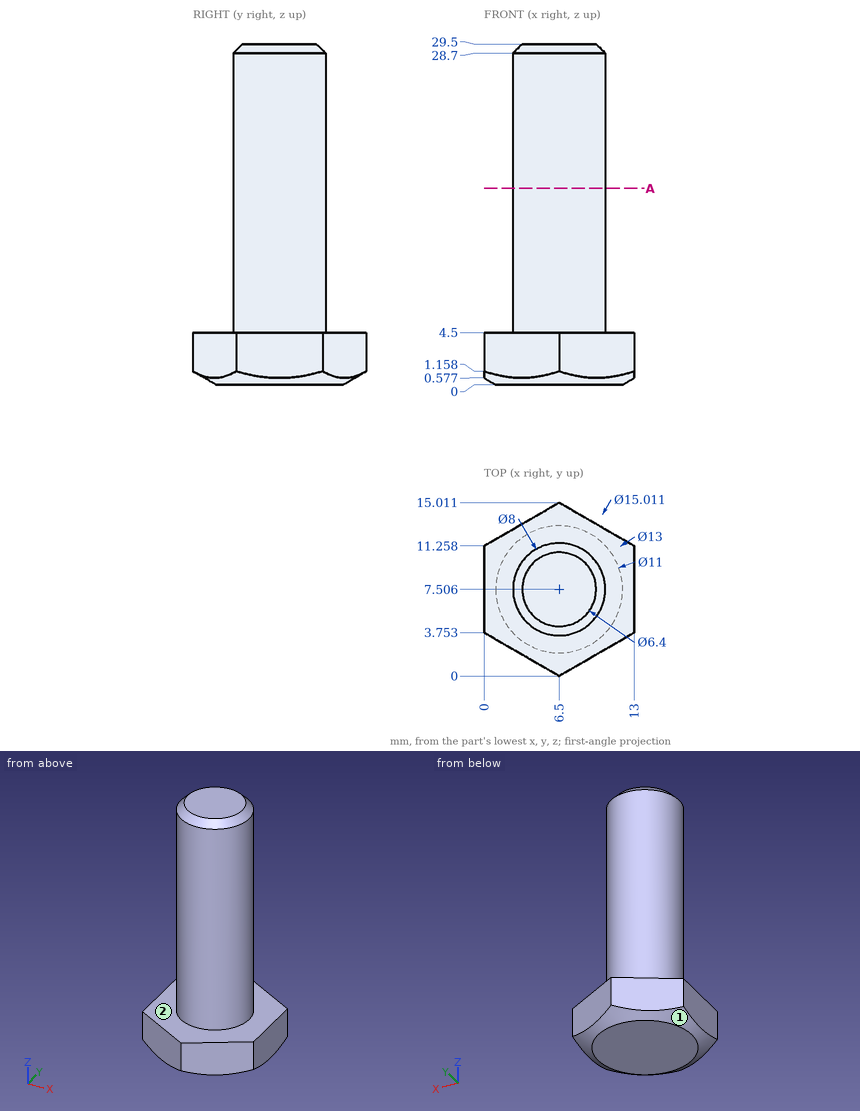
Check sheet for the drawn part. Datum: minimum x, y, z corner. Units: mm. A direction names the side the tool comes from. Give positions to 0.01 mm unless a question says otherwise; leave off trailing zeros. Order: outer loops, then holes, each group sorted by start corner. A loop starts at its lowest first (then second) coordinate and runs counter-clockwise, first axis right, second up. Notation, with made-up numbers: (-4, -32) -> (27, -32) arc R18 ccw to (27, -12) -> close; hole circle Ø6 at (51.25, 29). An arc over 180 degrees is marked (long way). Return JSON: item names as keys, results as strings.
1. Go/stop test with flat-tipped pins: P1, Ø3, axis at x = 8, z = 26, coming from the +Y side; P2, Ø1.5, axis at x = 8.5, z = 9.5, coming from the -Y side (1 decimal); P3, Ø4, axis at x = 2.5, y = 2.5, coming from the +Z side. Record where each tip stops, or that it passes through.
From the geometry:
{"P1": "y = 11.51", "P2": "y = 3.7", "P3": "z = 4.5"}
2. Material ranges on probe 1 along Z at (x, y) = (4.5, 11.5); probe 2 along X at (y, z) = (7.75, 22.5); probe 3 along Y at (x, z) = (6.5, 9) (1 decimal), recorded low to high. Write a range as [from, to].
From the geometry:
{"probe 1": "[0, 4.5]", "probe 2": "[2.51, 10.49]", "probe 3": "[3.5, 11.5]"}
3. Cross-section at A-A, the plane z = 17. Record the cut outline in (x, y) (1 decimal).
From the geometry:
{"outline": "circle Ø8 at (6.5, 7.5)"}
4. Set-up check for the marked faces 1 and 2: record each of +Z, -Z, +X, -X, +Y, -Y from which the full face is reachable in a straight line by a thin tool's end or side.
From the geometry:
{"face 1": "-Z", "face 2": "+Z"}
